Read the model definition and answer for the solid it produces. Units are mm, in the model's axes. A direction names the side the tool comes from. Round coordinates to 2 decimals unless told otherwise and drop trailing zeros. Write each loop counter-clockwise with the first axis right and the second up, starting at its lowest first coordinate (ties: lowest second). Pieces come first, ordered by that corner, then holes. Notation, with made-up numbers: (56, 80) -> (85, 80) arc R27 cw to (85, 112) -> close; hole circle Ø1 at (15.5, -3.75). An arc over 180 degrees is marked (long way). Return JSON: item names as keys, results as strings. Group by question number.
(1) For faces 1 (the cylindrical face through (11.25, 32.05, 26.2)), 2 (the flat face through (0, 20, 15)), 3 (the flat face through (26.96, 1.26, 15.21)), determine the directions among +Z, -Z, +X, -X, +Y, -Y from which every point of the face is accessible in a straight line to the end or side of a thin tool.
(2) A cutting plane is placed at B-B on x = 13. Give the vertices of the cut face in (y, z), then the cut area to 3 significant figures.
(3) Given pin 1 (1.5 mm diameter, centred on x = 30, y = 32, fed in from +Z); pin 2 (6.5 mm diameter, centred on x = 22, z = 9.5, fed in from -Y), each flat-ended and moving along its own axis, determine where each tip first touches the part or whether it passes through.
(4) Straight lines are drawn through the part: line 1 (Y direction, x = 10, z = 24.5); line 2 (Z direction, x = 20, y = 36); line 3 (Y direction, x = 17.5, z = 13.25). For each, find the intervals that lie inside material, in ascending order.
(5) A cutting plane is placed at A-A on z = 2.25. Give the vertices of the cut face in (x, y).
(6) The mould has two halves that part along Y. Classify faces 4 (the flat face through (5, 0, 15)), 5 (the cylindrical face through (22.5, 32.4, 14.9)), 6 (the flat face through (20, 40, 11)), 7 (the cylindrical face through (28.845, 31.521, 26.197)): released by +Y, released by -Y, zero draft, split by the parting line, or undercut.
```python
from build123d import *

# Parameters (mm, degrees)
SKETCH_1_W             = 40
SKETCH_1_H             = 40
EXTRUDE_1_DEPTH        = 30
CUT_EXTRUDE_1_DEPTH    = 65.031242374
HOLE_WIZARD_M6_1_D     = 5
HOLE_WIZARD_M6_1_DEPTH = 15
HOLE_WIZARD_M6_1_TIP   = 1.502151548
HOLE_WIZARD_M3_1_D     = 2.5
HOLE_WIZARD_M3_1_DEPTH = 7.5
HOLE_WIZARD_M3_1_TIP   = 0.751075774


with BuildPart() as part:
    # 草图1 → 凸台-拉伸1 (new body)
    with BuildSketch(Plane.XY):
        with Locations((20, 20)):
            Rectangle(SKETCH_1_W, SKETCH_1_H)
    extrude(amount=EXTRUDE_1_DEPTH)

    # 草图2 → 切除-拉伸1 (cut, through all)
    with BuildSketch(Plane.XY.offset(30)):
        Polygon((10, 0), (16, 2.485281374), (16, 4), (24, 4), (24, 2.485281374), (30, 0), align=None)
    extrude(amount=-CUT_EXTRUDE_1_DEPTH, mode=Mode.SUBTRACT)

    # M6 螺纹孔1
    with Locations(Plane(origin=(0, 40, 0), x_dir=(1, 0, 0), z_dir=(0, 1, 0))):
        with Locations((20, -15)):
            Hole(HOLE_WIZARD_M6_1_D / 2, depth=HOLE_WIZARD_M6_1_DEPTH)
            with Locations((0, 0, -(HOLE_WIZARD_M6_1_DEPTH + HOLE_WIZARD_M6_1_TIP / 2))):  # 118° drill point
                Cone(0, HOLE_WIZARD_M6_1_D / 2, HOLE_WIZARD_M6_1_TIP, mode=Mode.SUBTRACT)

    # M3 螺纹孔1
    with Locations(Plane.XY.offset(30)):
        with Locations((10, 32), (30, 32)):
            Hole(HOLE_WIZARD_M3_1_D / 2, depth=HOLE_WIZARD_M3_1_DEPTH)
            with Locations((0, 0, -(HOLE_WIZARD_M3_1_DEPTH + HOLE_WIZARD_M3_1_TIP / 2))):  # 118° drill point
                Cone(0, HOLE_WIZARD_M3_1_D / 2, HOLE_WIZARD_M3_1_TIP, mode=Mode.SUBTRACT)


solid = part.part
```
Checks:
{
 "1": {"face 1": "+Z", "face 2": "+Z, -Z, -X, +Y, -Y", "face 3": "+Z, -Z, -Y"},
 "2": {"outline": "(1.24, 0) -> (40, 0) -> (40, 30) -> (1.24, 30) -> close", "area": "1,160 mm^2"},
 "3": {"pin 1": "stops at z = 22.2", "pin 2": "stops at y = 1.97"},
 "4": {"line 1": "y = 0 to 30.75, 33.25 to 40", "line 2": "z = 0 to 12.5, 17.5 to 30", "line 3": "y = 4 to 40"},
 "5": {"outline": "(0, 0) -> (10, 0) -> (16, 2.49) -> (16, 4) -> (24, 4) -> (24, 2.49) -> (30, 0) -> (40, 0) -> (40, 40) -> (0, 40) -> close"},
 "6": {"face 4": "released by -Y", "face 5": "zero draft", "face 6": "released by +Y", "face 7": "undercut"}
}
